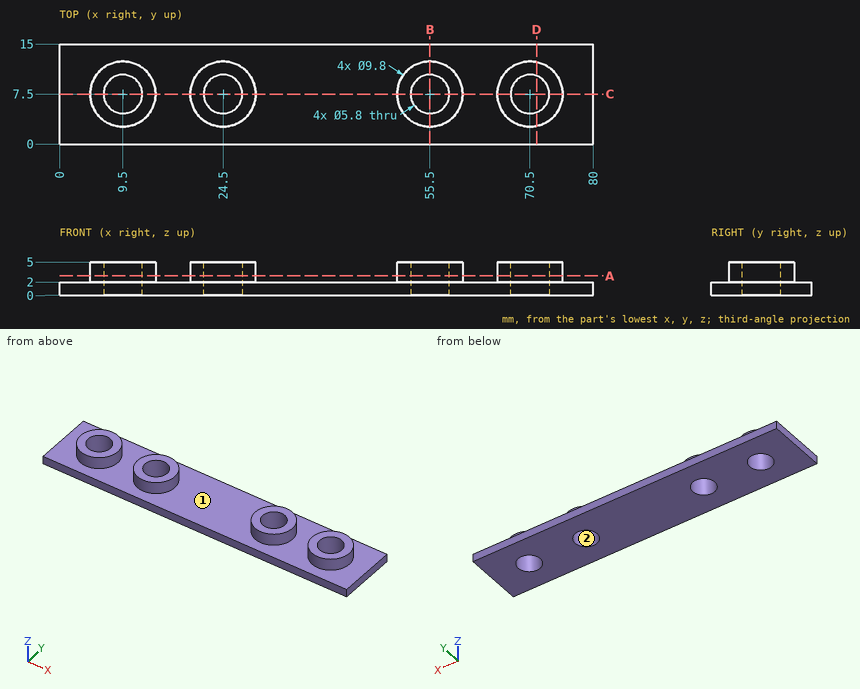
Can you work these out from the drawing? Everything is in mm from the part's minimum corner. Round coordinates to 2 decimals unless told otherwise and drop trailing zeros. Order: outer loops, then holes, each group sorted by start corner. A loop starts at its lowest first (then second) coordinate and runs counter-clockwise, first axis right, second up.
(1) If we section it at D-D (x = 71.5): Please give me the cut outline in (y, z).
Results are:
outline: (0, 0) - (4.78, 0) - (4.78, 5) - (2.7, 5) - (2.7, 2) - (0, 2) - close; (10.22, 0) - (15, 0) - (15, 2) - (12.3, 2) - (12.3, 5) - (10.22, 5) - close
(2) If we section it at C-C (y = 7.5): Count the separate pieces of the cut face and the enclosed holes in it, plus the area to 3 significant figures.
Results are:
separate pieces: 5
enclosed holes: 0
area: 162 mm2
(3) If we section it at B-B (x = 55.5): Please give me the cut outline in (y, z).
Results are:
outline: (0, 0) - (4.6, 0) - (4.6, 5) - (2.6, 5) - (2.6, 2) - (0, 2) - close; (10.4, 0) - (15, 0) - (15, 2) - (12.4, 2) - (12.4, 5) - (10.4, 5) - close
(4) If we section it at A-A (z = 2.95): Please give me the cut outline in (x, y).
Results are:
outline: circle Ø9.8 at (9.5, 7.5); circle Ø9.8 at (24.5, 7.5); circle Ø9.8 at (55.5, 7.5); circle Ø9.8 at (70.5, 7.5); hole circle Ø5.8 at (9.5, 7.5); hole circle Ø5.8 at (24.5, 7.5); hole circle Ø5.8 at (55.5, 7.5); hole circle Ø5.8 at (70.5, 7.5)
(5) If I drill on L1, parallel to Y at x = 9.5, z = 1.25; L2, parallel to Y at x = 9.5, z = 3.3; L3, parallel to X at y = 6, z = 0.8, over which ranges is the centre line in solid material (lowest first)?
Results are:
L1: y = 0 to 4.6, 10.4 to 15
L2: y = 2.6 to 4.6, 10.4 to 12.4
L3: x = 0 to 7.02, 11.98 to 22.02, 26.98 to 53.02, 57.98 to 68.02, 72.98 to 80
(6) We'd pull the mould along Y, two halves only. Please class the marked faces 1 and 2: +Y half, -Y half, draft (parallel to the pull), parting line (faces both ways), or undercut.
Results are:
face 1: draft
face 2: undercut
(7) I'm going to push a flat-ended pin straight in: pin 1 (4.5 mm diameter, centred on x = 70.5, y = 7.5, fed in from +Z). Where does the tip first touch, or does it pass through?
Results are:
pin 1: passes through
